Autodesk Inventor part; units mm, degrees
ref_plane "YZ Plane" through (0, 0, 0) normal (1, 0, 0) x (0, 1, 0)
ref_plane "XZ Plane" through (0, 0, 0) normal (0, 1, 0) x (-1, 0, 0)
ref_plane "XY Plane" through (0, 0, 0) normal (0, 0, 1) x (1, 0, 0)
sketch "Sketch1" plane through (0, 0, 0) normal (0, 0, 1) x (1, 0, 0)
  line L0 (-7.8232, 0) -> (7.8232, 0)
  line L1 (0, 7.8232) -> (0, -7.8232)
  line L2 (-5.588, 5.588) -> (5.588, 5.588)
  line L3 (5.588, 5.588) -> (5.588, -5.588)
  line L4 (5.588, -5.588) -> (-5.588, -5.588)
  line L5 (-5.588, -5.588) -> (-5.588, 5.588)
  point P0 (0, 0)
  point P1 (-5.588, 0)
  point P2 (0, 5.588)
  dimension "d0" = 11.176
  dimension "d1" = 11.176
extrude "Extrusion1" add sketch "Sketch1" along normal blind 3.81
sketch "Sketch2" plane through (0, 0, 3.81) normal (0, 0, 1) x (1, 0, 0)
  line L0 (-6.604, 6.604) -> (6.604, 6.604)
  line L1 (6.604, 6.604) -> (6.604, -6.604)
  line L2 (6.604, -6.604) -> (-6.604, -6.604)
  line L3 (-6.604, -6.604) -> (-6.604, 6.604)
  point P0 (0, 0)
  point P1 (-6.604, 0)
  point P2 (0, 6.604)
  dimension "d4" = 13.208
  dimension "d5" = 13.208
extrude "Extrusion2" add sketch "Sketch2" along normal blind 4.445
sketch "Sketch3" plane through (0, 0, 0) normal (0, 0, 1) x (1, 0, 0)
  line L0 (-4.7625, 4.7625) -> (4.7625, 4.7625)
  line L1 (4.7625, 4.7625) -> (4.7625, -4.7625)
  line L2 (4.7625, -4.7625) -> (-4.7625, -4.7625)
  line L3 (-4.7625, -4.7625) -> (-4.7625, 4.7625)
  point P0 (0, 0)
  point P1 (-4.7625, 0)
  point P2 (0, 4.7625)
  dimension "d8" = 9.525
  dimension "d9" = 9.525
extrude "Extrusion3" cut sketch "Sketch3" along normal through all
sketch "Sketch4" plane through (0, 0, 8.255) normal (0, 0, 1) x (1, 0, 0)
  line L0 (-0.7937, 6.0008) -> (0.7937, 6.0008)
  line L1 (0.7937, 6.0008) -> (0.7937, -6.0008)
  line L2 (0.7937, -6.0008) -> (-0.7937, -6.0008)
  line L3 (-0.7937, -6.0008) -> (-0.7937, 6.0008)
  point P0 (0, 0)
  point P1 (-0.7938, 0)
  point P2 (0, 6.0008)
  dimension "d14" = 12.0015
  dimension "d15" = 1.5875
extrude "Extrusion4" cut sketch "Sketch4" against normal blind 1.778
fillet "Fillet1" radius 2.3813 4 edges at (-4.7625, 4.7625, 4.1275) (4.7625, 4.7625, 4.1275) (4.7625, -4.7625, 4.1275) (-4.7625, -4.7625, 4.1275)
fillet "Fillet2" radius 3.302 8 edges at (-5.588, -5.588, 1.905) (-5.588, 5.588, 1.905) (5.588, -5.588, 1.905) (5.588, 5.588, 1.905) (-6.604, 6.604, 6.0325) (-6.604, -6.604, 6.0325) (6.604, -6.604, 6.0325) (6.604, 6.604, 6.0325)
fillet "Fillet3" radius 0.508 4 edges at (0.7937, 6.0008, 7.366) (-0.7937, 6.0008, 7.366) (-0.7937, -6.0008, 7.366) (0.7937, -6.0008, 7.366)
chamfer "Chamfer1" distance 0.508 angle 60 8 edges at (4.065, 4.065, 0) (4.7625, 0, 0) (4.065, -4.065, 0) (0, -4.7625, 0) (-4.065, -4.065, 0) (-4.7625, 0, 0) (-4.065, 4.065, 0) (0, 4.7625, 0) measured on face at (0.762, 5.0377, 0)
equation "\"d9\" = d8"
properties part number "J002873" material "ALUMINUM, 6061-T651"
CAD build for the part. Positions are in the model's coordinates, mm. A direction names the side the tool comes from. Give positions to 0.01 mm unless a question says otherwise; leave off trailing zeros. Write each loop counter-clockwise with the first axis right and the second up, starting at its lowest first coordinate (ties: lowest second). Pieces come first, ordered by that corner, then holes. Notation, with made-up numbers: M -9.5,-4 L 18.5,-4 A27 cw 18.5,34 Z; hole C -6,35.5 d6. An arc over 180 degrees is marked long. Put each result on its own line as item: value. Start each with the question number.
(1) Band-saw the part on D-D, the plane z = 7. Write the cut outline in (x, y).
(2) Band-saw the part on B-B, the plane z = 1.75. Write the cut outline in (x, y), and give its area (3 significant figures).
(3) Flat gauge pins, fed straight in: pin 1 Ø1.9 at (x, z) = (0, 1.5) entering from -Y; pin 2 Ø1.9 at (y, z) = (0, 2.5) entering from +X; pin 3 Ø0.6 at (y, z) = (5, 7) entering from -X. Where does each tip first touch, or does it go through?
(4) Probe L1, parallel to X at y = 0.25, z = 6.25; L2, parallel to X at y = -1, z = 2.5. List the from-to ranges inside material, lowest first.
(5) Which spindle directions (+Z, -Z, +X, -X, +Y, -Y) get a long thin tool onto all of the face, cutting with end or side? Do faces 1 (the face through (5.588, 0, 2)), 2 (the face through (0, -5.588, 2)), 3 (the face through (-4.08, -4.05, 4.62)), 4 (the face through (4.595, -4.646, 1.932)), 5 (the face through (4.187, 4.227, 0.532)). Say none if no direction does.
Response values:
1. outline: M -6.6,-3.3 A3.3 ccw -3.3,-6.6 L 3.3,-6.6 A3.3 ccw 6.6,-3.3 L 6.6,3.3 A3.3 ccw 3.3,6.6 L -3.3,6.6 A3.3 ccw -6.6,3.3 Z; hole M -4.76,-2.38 A2.38 ccw -2.38,-4.76 L -0.79,-4.76 L -0.79,-5.49 A0.51 ccw -0.29,-6 L 0.29,-6 A0.51 ccw 0.79,-5.49 L 0.79,-4.76 L 2.38,-4.76 A2.38 ccw 4.76,-2.38 L 4.76,2.38 A2.38 ccw 2.38,4.76 L 0.79,4.76 L 0.79,5.49 A0.51 ccw 0.29,6 L -0.29,6 A0.51 ccw -0.79,5.49 L -0.79,4.76 L -2.38,4.76 A2.38 ccw -4.76,2.38 Z
2. outline: M -5.59,-2.29 A3.3 ccw -2.29,-5.59 L 2.29,-5.59 A3.3 ccw 5.59,-2.29 L 5.59,2.29 A3.3 ccw 2.29,5.59 L -2.29,5.59 A3.3 ccw -5.59,2.29 Z; hole M -4.76,-2.38 A2.38 ccw -2.38,-4.76 L 2.38,-4.76 A2.38 ccw 4.76,-2.38 L 4.76,2.38 A2.38 ccw 2.38,4.76 L -2.38,4.76 A2.38 ccw -4.76,2.38 Z
2. area: 29.7 mm2
3. pin 1: stops at y = -5.59
3. pin 2: stops at x = 5.59
3. pin 3: stops at x = -6.29
4. L1: x = -6.6 to -4.76, 4.76 to 6.6
4. L2: x = -5.59 to -4.76, 4.76 to 5.59
5. face 1: -Z, +X, +Y, -Y
5. face 2: -Z, +X, -X, -Y
5. face 3: +Z, -Z
5. face 4: -Z, +X, -Y
5. face 5: -Z
